Autodesk Inventor part; units mm, degrees
ref_plane "nt_XY" through (0, 0, 0) normal (1, 0, 0) x (0, 0, -1)
ref_plane "nt_YZ" through (0, 0, 0) normal (0, 0, -1) x (0, 1, 0)
ref_plane "nt_ZX" through (0, 0, 0) normal (0, 1, 0) x (1, 0, 0)
sketch "B" plane through (0, 0, 0) normal (1, 0, 0) x (0, 1, 0)
  line L0 (-2.3094, 4) -> (-4.6188, 0)
  line L1 (-4.6188, 0) -> (-2.3094, -4)
  line L2 (-2.3094, -4) -> (2.3094, -4)
  line L3 (2.3094, -4) -> (4.6188, 0)
  line L4 (4.6188, 0) -> (2.3094, 4)
  line L5 (2.3094, 4) -> (-2.3094, 4)
extrude "Extrusion1" add sketch "B" along normal mid plane 4
sketch "Sketch_2" plane through (0, 0, 0) normal (0, 0, 1) x (1, 0, 0)
  line L0 (2, 0) -> (-2, 0)
  line L1 (-2, 0) -> (-2, 2.5)
  line L2 (-2, 2.5) -> (-1.567, 2.067)
  line L3 (-1.567, 2.067) -> (1.567, 2.067)
  line L4 (1.567, 2.067) -> (2, 2.5)
  line L5 (2, 2.5) -> (2, 0)
  line L6 (2, 0) -> (-2, 0)
revolve "Revolution1" cut sketch "Sketch_2" angle 360 about axis through (2, 0, 0) along (1, 0, 0)
thread "Thread1"
sketch "Sketch_3" plane through (0, 0, 0) normal (0, 0, 1) x (1, 0, 0)
  line L0 (50, 0) -> (-50, 0)
  line L1 (-7, 1) -> (-2, 1)
  line L2 (-2, 1) -> (-2, 3.44)
  line L3 (-2, 3.44) -> (0, 6.9041)
  line L4 (0, 6.9041) -> (2, 3.44)
  line L5 (2, 3.44) -> (2, 1)
  line L6 (2, 1) -> (7, 1)
  line L7 (7, 1) -> (7, 8.44)
  line L8 (7, 8.44) -> (-7, 8.44)
  line L9 (-7, 8.44) -> (-7, 1)
revolve "Revolution2" cut sketch "Sketch_3" angle 360 about axis through (50, 0, 0) along (1, 0, 0)
ref_plane "nt_XY" through (0, 0, 0) normal (1, 0, 0) x (0, 0, -1)
ref_plane "nt_YZ" through (0, 0, 0) normal (0, 0, -1) x (0, 1, 0)
ref_plane "nt_ZX" through (0, 0, 0) normal (0, 1, 0) x (1, 0, 0)
ref_plane "ntj_XY" through (2, 0, 0) normal (1, 0, 0) x (0, 0, -1)
ref_plane "ntj_YZ" through (2, 0, 0) normal (0, 0, -1) x (0, 1, 0)
ref_plane "ntj_ZX" through (2, 0, 0) normal (0, 1, 0) x (1, 0, 0)
properties part number "NTJ-015C"
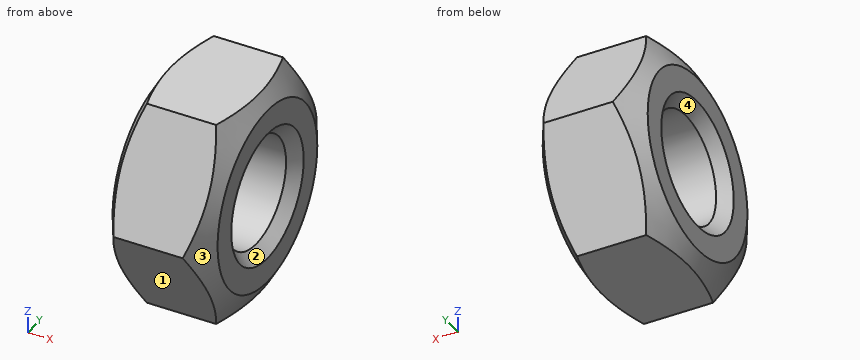
Part model, mm, in its own coordinate system. Face numbers are marked on the shaded views. Coordinates: 2 decimals unless noted, no trailing zeros. Write each loop counter-clockwise with the first axis right and the second up, starting at its lowest first coordinate (ties: lowest second). Pieces come first, ordered by that corner, then holes.
Item 1: Probe line 1 (Z direction, x = -0.3, y = 0); line 2 (Z direction, x = 0.05, y = -0.5); line 3 (Y direction, x = 0.6, z = -1.5). List the from-to ranges inside material, lowest first.
Item 2: Mould opens along Y. For the marked faces 1, 2, 3 and 4 say: released by +Y, released by -Y, zero draft, split by the parting line, or undercut.
Item 3: Slice it at A-A (x = 0.8). Write the cut outline in (y, z).
Item 4: Slice it at B-B (y = 0). Write the cut outline in (x, z).
Item 5: Pin check, flat tips, straight feed: pin 1 (1 mm diameter, centred on x = 0, y = 3, fed in from +Z); pin 2 (2 mm diameter, centred on x = 0, z = -3, fed in from -Y); pin 3 (1.5 mm diameter, centred on x = 1, z = 2, fed in from +Y). Stop position of each tip, or through.
Results found:
1. line 1: z = -4 to -2.07, 2.07 to 4
1. line 2: z = -4 to -2.01, 2.01 to 4
1. line 3: y = -3.75 to -1.42, 1.42 to 3.75
2. face 1: released by -Y
2. face 2: undercut
2. face 3: split by the parting line
2. face 4: undercut
3. outline: (-4.62, 0) - (-2.31, -4) - (2.31, -4) - (4.62, 0) - (2.31, 4) - (-2.31, 4) - close; hole circle Ø4.13 at (0, 0)
4. outline: (-2, -3.44) - (-1.68, -4) - (1.68, -4) - (2, -3.44) - (2, -2.5) - (1.57, -2.07) - (-1.57, -2.07) - (-2, -2.5) - close; (-2, 2.5) - (-1.57, 2.07) - (1.57, 2.07) - (2, 2.5) - (2, 3.44) - (1.68, 4) - (-1.68, 4) - (-2, 3.44) - close
5. pin 1: stops at z = 3.67
5. pin 2: stops at y = -3.46
5. pin 3: stops at y = 3.9
